from build123d import *

# Parameters (mm, degrees)
F1_DEPTH        = 12
F2_R            = 9
F3_R            = 5
F4_R            = 9
F5_R            = 5
F6_R            = 5
F7_R            = 5
F8_T1_DEPTH     = 30
F10_R           = 5
F11_R           = 9
F13_D           = 4
F13_CSINK_D     = 5
F13_CSINK_ANGLE = 45
F14_D           = 4
F14_CSINK_D     = 5
F14_CSINK_ANGLE = 45


# Not quite as in the source:
# - a fillet or chamfer that OpenCascade refuses, or shapes differently, is made with other operations: its cross-section is extruded or revolved along the edge and cut away or added


with BuildPart() as f1:
    # F0 (on Front) → F1 (new body)
    with BuildSketch(Plane.XZ):
        Polygon((0, 40.3702630328), (0, 0), (20.5587926316, 0), (25.9716099992, 9.9235005083), (21.5821319316, 12.3177607896), (17.5906268513, 5), (5, 5), (5, 37.6631405767), (43.3543724833, 62.7000143926), (40.621260608, 66.8869105553), align=None)
    extrude(amount=F1_DEPTH)

    # F2
    f2_edges = [f1.edges().sort_by_distance(p)[0] for p in [
        (20.558793, -6, 0),
    ]]
    fillet(f2_edges, radius=F2_R)

    # F3
    f3_edges = [f1.edges().sort_by_distance(p)[0] for p in [
        (17.590627, -6, 5),
    ]]
    fillet(f3_edges, radius=F3_R)

    # F4
    f4_edges = [f1.edges().sort_by_distance(p)[0] for p in [
        (0, -6, 40.370263),
    ]]
    fillet(f4_edges, radius=F4_R)

    # F5
    f5_edges = [f1.edges().sort_by_distance(p)[0] for p in [
        (5, -6, 37.663141),
    ]]
    fillet(f5_edges, radius=F5_R)

    # F6
    f6_edges = [f1.edges().sort_by_distance(p)[0] for p in [
        (23.776871, -12, 11.120631),
    ]]
    fillet(f6_edges, radius=F6_R)

    # F7
    f7_edges = [f1.edges().sort_by_distance(p)[0] for p in [
        (23.776871, 0, 11.120631),
    ]]
    fillet(f7_edges, radius=F7_R)

    # F8: fillet of radius 5 on 2 edges, made by hand

    # F8_s2 → F8_t1 (cut)
    with BuildSketch(Plane(origin=(-8.9127980143, 0, 13.6536525057), x_dir=(0, 1, 0), z_dir=(-0.5466223751, 0, 0.8373792325))):
        with BuildLine():
            add(Edge.make_bspline(
                [(-12, -65.577281941), (-12, -70.577281941), (-7, -70.577281941)],
                knots=[0, 0, 0, 1, 1, 1], degree=2, weights=[1, 1, 1]))
            Line((-7, -70.577281941), (-12, -70.577281941))
            Line((-12, -70.577281941), (-12, -65.577281941))
        make_face()
        with BuildLine():
            add(Edge.make_bspline(
                [(0, -65.577281941), (0, -70.577281941), (-5, -70.577281941)],
                knots=[0, 0, 0, 1, 1, 1], degree=2, weights=[1, 1, 1]))
            Line((-5, -70.577281941), (0, -70.577281941))
            Line((0, -70.577281941), (0, -65.577281941))
        make_face()
    extrude(amount=F8_T1_DEPTH, mode=Mode.SUBTRACT)

    # F10
    f10_edges = [f1.edges().sort_by_distance(p)[0] for p in [
        (5, -6, 5),
    ]]
    fillet(f10_edges, radius=F10_R)

    # F11
    f11_edges = [f1.edges().sort_by_distance(p)[0] for p in [
        (0, -6, 0),
    ]]
    fillet(f11_edges, radius=F11_R)

    # F13 (through all)
    with Locations(Plane.YZ.offset(5)):
        with Locations((-8.210901171, 27.0586498082)):
            CounterSinkHole(F13_D / 2, F13_CSINK_D / 2, counter_sink_angle=F13_CSINK_ANGLE)

    # F14 (through all)
    with Locations(Plane.YZ.offset(5)):
        with Locations((-4.1054510511, 18.6611376703)):
            CounterSinkHole(F14_D / 2, F14_CSINK_D / 2, counter_sink_angle=F14_CSINK_ANGLE)


solid = f1.part
The listing builds one solid part. Answer for the finished solid, in the listing's coordinates (mm). A direction names the side the tool comes from. Give positions to 0.01 mm unless a question says otherwise; leave off trailing zeros. Write each loop counter-clockwise with the first axis right and the second up, starting at its lowest first coordinate (ties: lowest second). Pieces come first, ordered by that corner, then holes.
Item 1: Which of the six approach directions +Z, -Z, +X, -X, +Y, -Y give full straight-line access (tool end or side, diameter ignored) to faces 5 (the cylindrical face through (17.21, -6.08, 5.72)), 6 (the cylindrical face through (23.063, -10.496, 9.886)), 7 (the flat face through (24, -6, 11))?
Item 2: Section B-B, the plane z = 33 is taken. Write down the section's boundary in (x, y), plus the area to 3 significant figures.
Item 3: Section C-C, the plane x = 6.5 is taken. Write down the section's boundary in (y, z).
Item 4: Find the intervals of material crossed by line 1 along X through (y, z) = (-9.75, 13); line 2 along Z through (x, y) = (3, -5.5); line 3 along Z through (x, y) = (11.5, -9.75), in increasing order.
Item 5: Section D-D, the plane z = 57.5 is taken. Write down the section's boundary in (x, y).
Item 6: Determine the mould class of faces 1 (the flat face through (12, -6, 5)), 2 (the cylindrical face through (6, -6, 7)), 3 (the flat face through (25.06, -5.92, 50.76)), 4 (the flat face through (4, -12, 27)) for opening direction X: released by +X, released by -X, zero draft, split by the parting line, or undercut.
Item 7: Flat-ended cylindrical pins translate along their axes: P1, Ø2, axis at y = -7.5, z = 41.5, coming from the -X side; P2, Ø3, axis at x = 25.5, y = -8.5, coming from the -Z side; P3, Ø3.5, axis at x = 11.5, y = -3, coming from the +Z side; P4, Ø3, axis at y = -8.21, z = 27.06, coming from the -X side. Find the tip coordinate at first contact, or state that the pin passes through.
Item 8: Section A-A, the plane x = 16 is taken. Write down the section's boundary in (y, z).
Completed:
1. face 5: +Y, -Y
1. face 6: +X, -Y
1. face 7: +X, +Y, -Y
2. outline: (0, -12) - (5, -12) - (5, 0) - (0, 0) - close
2. area: 60.0 mm2
3. outline: (-12, 0.35) - (0, 0.35) - (0, 6.43) - (-12, 6.43) - close; (-12, 38.53) - (0, 38.53) - (0, 44.61) - (-12, 44.61) - close
4. line 1: x = 0 to 5
4. line 2: z = 2.29 to 17.23, 20.09 to 42.21
4. line 3: z = 0 to 5, 41.91 to 47.88
5. outline: (26.24, -12) - (35.39, -12) - (35.39, 0) - (26.24, 0) - close
6. face 1: undercut
6. face 2: undercut
6. face 3: released by +X
6. face 4: zero draft
7. P1: stops at x = 1.52
7. P2: stops at z = 6.31
7. P3: stops at z = 49.02
7. P4: passes through
8. outline: (-12, 0.03) - (0, 0.03) - (0, 5.19) - (-12, 5.19) - close; (-12, 44.84) - (0, 44.84) - (0, 50.81) - (-12, 50.81) - close
